Geometry: see drawing. Coordinates: mm, zero at the bounding-box minimum. A direction names the side the tool comes from. Coordinates: 2 decimals unless noted, no trailing zeros. Write each loop counter-clockwise with the first axis right and the second up, starting at its lowest first coordinate (ties: lowest second). Pieces come first, ordered by that corner, then holes. Notation, with made-up numbers: (70, 33.25) - (105, 33.25) arc R34 cw to (105, 69.25) - close; hole circle Ø4 at (28.5, 16.5). An arc over 180 degrees is marked (long way). One line per question, with ' | ' between items. Start each with the question number.
1) First-contact query: P1, Ø4, axis at x = 76.5, z = 130, coming from the -Y side; P2, Ø4, axis at x = 78.5, z = 148, coming from the -Y side. Flat tips, straight axial feed; report the tip coordinate or a pass-through.
2) Line query: line 1 (X direction, y = 23.5, z = 95); line 2 (Y direction, x = 86.5, z = 34.5). Output: solid intervals per line, ascending.
3) Section query C-C on x = 45. Return loops of the section in (y, z).
4) Reachability of the marked faces 1 and 2 from +Z, -Z, +X, -X, +Y, -Y: full face, straight path, thin tool, end or side. Return the list, or none.
5) Section query A-A on y = 79. Return loops of the section in (x, z).
6) Draft query along Z for the marked faces 3, 4, 5 and 6. Return one class per face: released by +Z, released by -Z, zero draft, split by the parting line, or undercut.
7) Section query B-B on z = 12. Return loops of the section in (x, y).
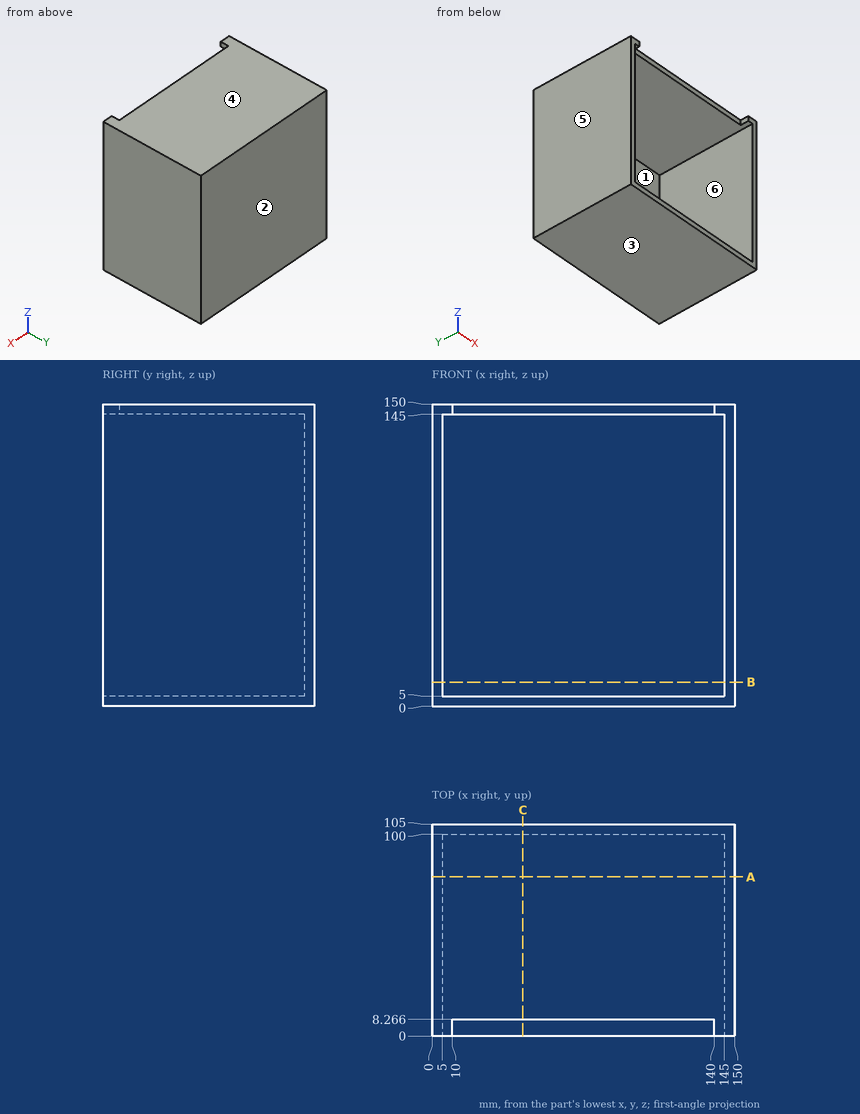
Answer key:
1) P1: y = 100 | P2: y = 8.27
2) line 1: 0 to 5, 145 to 150 | line 2: 100 to 105
3) outline: (0, 0) - (105, 0) - (105, 150) - (8.27, 150) - (8.27, 145) - (100, 145) - (100, 5) - (0, 5) - close
4) face 1: -Y | face 2: +Z, -Z, +X, -X, +Y
5) outline: (0, 0) - (150, 0) - (150, 150) - (0, 150) - close; hole (5, 5) - (145, 5) - (145, 145) - (5, 145) - close
6) face 3: released by -Z | face 4: released by +Z | face 5: zero draft | face 6: undercut
7) outline: (0, 0) - (5, 0) - (5, 100) - (145, 100) - (145, 0) - (150, 0) - (150, 105) - (0, 105) - close
